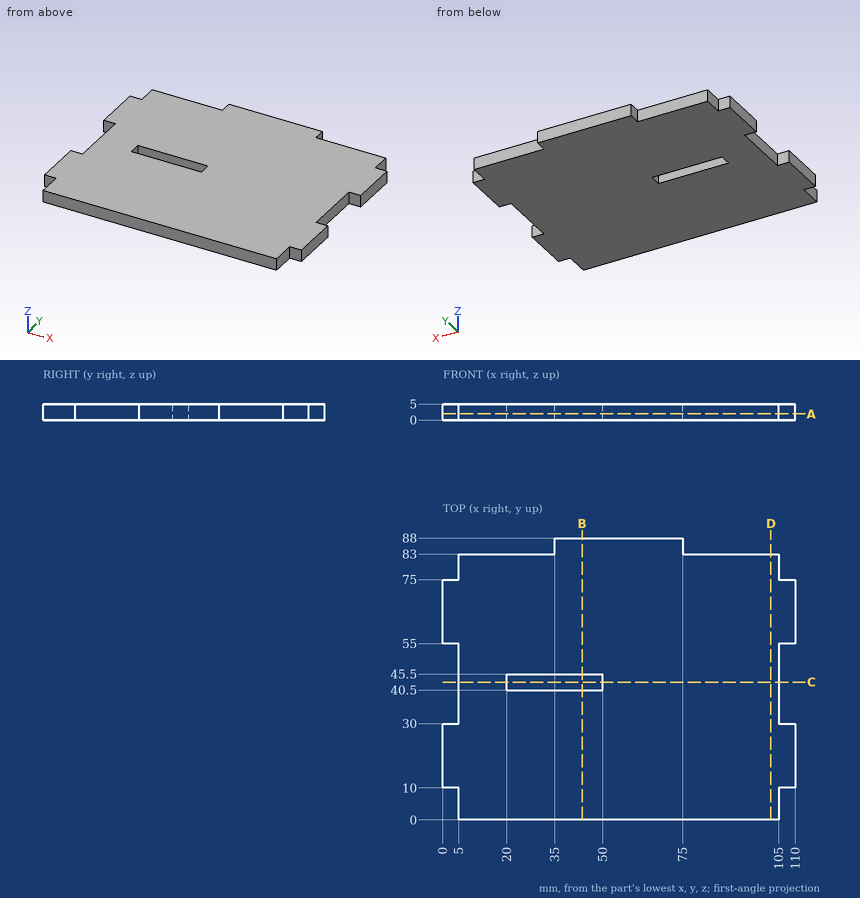
Input: dimensioned drawing with shaded views. Units: mm. Origin: part minimum x, y, z. Coordinates: 2 decimals unless noted, no trailing zeros. Write each loop counter-clockwise with the first axis right and the second up, starting at its lowest first coordinate (ties: lowest second). Pieces come first, ordered by that corner, then holes. Notation, with made-up numbers: M -29.5,-23.75 L 23.5,-23.75 A24 ccw 23.5,-4.75 Z; hole C -40,27 d8. An arc over 180 degrees is marked long. Answer as a JSON object with one key per item and string values. Group by question number.
(1) Section B-B on x = 43.5. Output: boundary loops of the cut face in (y, z), plus the area to 3 significant figures.
(2) Section C-C on y = 43. Output: boundary loops of the cut face in (x, z).
(3) Section A-A on z = 1.9. Output: boundary loops of the cut face in (x, y), plus the area to 3 significant figures.
(4) Contact query for flat-ended pins moving along their axis: P1, Ø1, axis at x = 77.5, y = 27.5, coming from the -Z side; P2, Ø1, axis at y = 33, z = 1.5, coming from the +X side; P3, Ø1.5, axis at x = 92.5, z = 1.5, coming from the +Y side; P4, Ø1.5, axis at x = 106.5, z = 1.5, coming from the +Y side. Output: stop coordinate, or through.
(5) Ray query, line 1 along Y through (x, z) = (41.5, 4.3); line 2 along Y through (x, z) = (105.5, 2.5); line 3 along X through (y, z) = (44.5, 1.9). Return the intervals inside material, ascending. Write a range as [from, to].
(6) Section D-D on x = 102.5. Output: boundary loops of the cut face in (y, z).
Result set:
{
 "1": {"outline": "M 0,0 L 40.5,0 L 40.5,5 L 0,5 Z; M 45.5,0 L 88,0 L 88,5 L 45.5,5 Z", "area": "415 mm2"},
 "2": {"outline": "M 5,0 L 20,0 L 20,5 L 5,5 Z; M 50,0 L 105,0 L 105,5 L 50,5 Z"},
 "3": {"outline": "M 0,10 L 5,10 L 5,0 L 105,0 L 105,10 L 110,10 L 110,30 L 105,30 L 105,55 L 110,55 L 110,75 L 105,75 L 105,83 L 75,83 L 75,88 L 35,88 L 35,83 L 5,83 L 5,75 L 0,75 L 0,55 L 5,55 L 5,30 L 0,30 Z; hole M 20,40.5 L 50,40.5 L 50,45.5 L 20,45.5 Z", "area": "8,750 mm2"},
 "4": {"P1": "stops at z = 0", "P2": "stops at x = 105", "P3": "stops at y = 83", "P4": "stops at y = 75"},
 "5": {"line 1": "y = [0, 40.5], [45.5, 88]", "line 2": "y = [10, 30], [55, 75]", "line 3": "x = [5, 20], [50, 105]"},
 "6": {"outline": "M 0,0 L 83,0 L 83,5 L 0,5 Z"}
}
